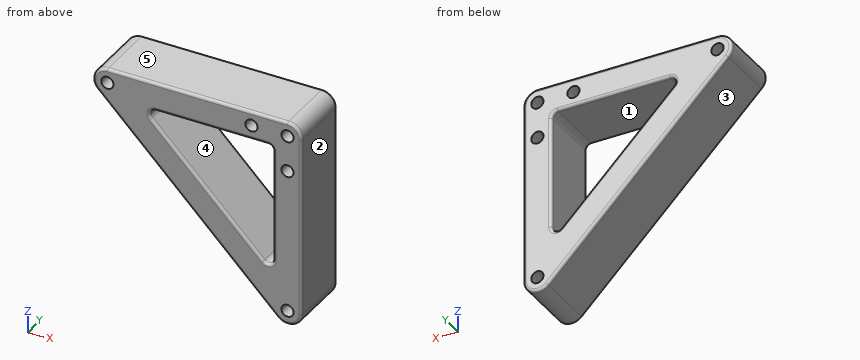
from build123d import *

# Parameters (mm, degrees)
SKETCH1_R           = 2.15
BOSS_EXTRUDE1_DEPTH = 22.2504
FILLET1_R           = 5
FILLET2_R           = 2
FILLET3_R           = 1


with BuildPart() as part:
    # Sketch1 → Boss-Extrude1 (new body)
    with BuildSketch(Plane(origin=(0, 0, 0), x_dir=(1, 0, 0), z_dir=(0, 1, 0))):
        with BuildLine():
            Line((59.964466094, 67.035533906), (-3.535533906, 3.535533906))
            ThreePointArc((-3.535533906, 3.535533906), (-4.619397663, -1.913417162), (0, -5))
            Line((0, -5), (68.5, -5))
            Line((68.5, -5), (68.5, 63.5))
            ThreePointArc((68.5, 63.5), (65.413417162, 68.119397663), (59.964466094, 67.035533906))
        make_face()
        Polygon((12.071067812, 5), (58.5, 51.428932188), (58.5, 5), align=None, mode=Mode.SUBTRACT)
        with Locations(Location((0, 0, 0), (0, 0, 90))):
            Circle(SKETCH1_R, mode=Mode.SUBTRACT)
        with Locations(Location((63.5, 63.5, 0), (0, 0, 90))):
            Circle(SKETCH1_R, mode=Mode.SUBTRACT)
        with Locations(Location((50.8, 0, 0), (0, 0, 90))):
            Circle(SKETCH1_R, mode=Mode.SUBTRACT)
        with Locations(Location((63.5, 0, 0), (0, 0, 90))):
            Circle(SKETCH1_R, mode=Mode.SUBTRACT)
        with Locations(Location((63.5, 12.7, 0), (0, 0, 90))):
            Circle(SKETCH1_R, mode=Mode.SUBTRACT)
    extrude(amount=BOSS_EXTRUDE1_DEPTH)

    # Fillet1
    fillet1_edges = [part.edges().sort_by_distance(p)[0] for p in [
        (68.5, 11.1252, 5),
    ]]
    fillet(fillet1_edges, radius=FILLET1_R)

    # Fillet2
    fillet2_edges = [part.edges().sort_by_distance(p)[0] for p in [
        (58.5, 11.1252, -5),
        (58.5, 11.1252, -51.428932188),
        (12.071067812, 11.1252, -5),
    ]]
    fillet(fillet2_edges, radius=FILLET2_R)

    # Fillet3
    fillet3_edges = [part.edges().sort_by_distance(p)[0] for p in [
        (68.5, 22.2504, -31.75),
        (65.413417162, 22.2504, -68.119397663),
        (31.75, 0, 5),
        (-4.619397663, 0, 1.913417162),
        (28.214466094, 22.2504, -35.285533906),
        (28.214466094, 0, -35.285533906),
        (65.413417162, 0, -68.119397663),
        (68.5, 0, -31.75),
        (-4.619397663, 22.2504, 1.913417162),
        (31.75, 22.2504, 5),
        (67.035533906, 0, 3.535533906),
        (67.035533906, 22.2504, 3.535533906),
        (58.5, 0, -26.800252532),
        (58.5, 22.2504, -26.800252532),
        (35.285533906, 0, -28.214466094),
        (35.285533906, 22.2504, -28.214466094),
        (36.699747468, 0, -5),
        (36.699747468, 22.2504, -5),
        (57.265366865, 0, -48.448264128),
        (57.265366865, 22.2504, -48.448264128),
        (57.914213562, 0, -5.585786438),
        (57.914213562, 22.2504, -5.585786438),
        (15.051735872, 0, -6.234633135),
        (15.051735872, 22.2504, -6.234633135),
    ]]
    fillet(fillet3_edges, radius=FILLET3_R)


solid = part.part
Check sheet for the modelled part. Datum: model origin and axes. Units: mm. Face numbers are marked on the shaded views. A direction names the side the tool comes from. Round coordinates to 2 decimals unless told otherwise and drop trailing zeros. Loops run counter-clockwise (first coordinate to the right, second up) from the corner with the lowest first, then second, coordinate; pieces in that order, holes last.
1. Scan lines: probe 1 along X at (y, z) = (17.25, 0); probe 2 along Z at (x, y) = (63.5, 5.25); probe 3 along X at (y, z) = (12, -12.7). Record each from-to range of solid material in increasing order.
2. Sectioned sample at A-A on y = 14.75. Record the boundary of the cut face in (x, z), and give its area (3 significant figures).
3. Sectioned sample at B-B on x = 50.8. Give the number of separate pieces and of enclosed holes in the cut face, and give its area (3 significant figures).
4. Gauge pin test, flat ends, axial feed: pin 1 Ø2 at (x, y) = (36.5, 12.5) entering from -Z; pin 2 Ø1 at (x, y) = (26, 20) entering from -Z; pin 3 Ø3 at (y, z) = (3.5, -5.5) entering from -X. Record the tip position at first contact, or that the pin passes through.
5. Set-up check for the marked faces 4 and 5: record each of +Z, -Z, +X, -X, +Y, -Y from which the full face is reachable in a straight line by a thin tool's end or side.
6. Mould release check, pull along X, two halves, no side actions. Record for the marked faces 1, 2 and 3: released by +X, released by -X, zero draft, split by the parting line, or undercut.
Recorded:
1. probe 1: x = -5 to -2.15, 2.15 to 48.65, 52.95 to 61.35, 65.65 to 68.5
1. probe 2: z = -68.5 to -65.65, -61.35 to -14.85, -10.55 to -2.15, 2.15 to 5
1. probe 3: x = 5.63 to 19.77, 58.5 to 61.35, 65.65 to 68.5
2. outline: (-3.54, -3.54) - (59.96, -67.04) arc R5 ccw to (68.5, -63.5) - (68.5, 0) arc R5 ccw to (63.5, 5) - (0, 5) arc R5 ccw to start; hole circle Ø4.3 at (0, 0); hole (15.49, -8.41) - (55.09, -48.01) arc R2 ccw to (58.5, -46.6) - (58.5, -7) arc R2 ccw to (56.5, -5) - (16.9, -5) arc R2 ccw to start; hole circle Ø4.3 at (50.8, 0); hole circle Ø4.3 at (63.5, -63.5); hole circle Ø4.3 at (63.5, -12.7); hole circle Ø4.3 at (63.5, 0)
2. area: 2,040 mm2
3. separate pieces: 3
3. enclosed holes: 0
3. area: 439 mm2
4. pin 1: stops at z = -44.57
4. pin 2: stops at z = -33.57
4. pin 3: stops at x = -3.07
5. face 4: +Y, -Y
5. face 5: +Z, +X, -X, +Y, -Y
6. face 1: undercut
6. face 2: released by +X
6. face 3: released by -X
